```python
from build123d import *

# Parameters (mm, degrees)
EXTRUDE_1_DEPTH     = 6
SKETCH_2_R          = 2
CUT_EXTRUDE_1_DEPTH = 81.380345856


with BuildPart() as part:
    # 草图1 → 凸台-拉伸1 (new body)
    with BuildSketch(Plane(origin=(0, 0, 0), x_dir=(0, 0, -1), z_dir=(1, 0, 0))):
        with BuildLine():
            Line((0, 5), (75, 5))
            ThreePointArc((75, 5), (80, 0), (75, -5))
            Line((75, -5), (0, -5))
            ThreePointArc((0, -5), (-5, 0), (0, 5))
        make_face()
    extrude(amount=EXTRUDE_1_DEPTH)

    # 草图2 → 切除-拉伸1 (cut, through all)
    with BuildSketch(Plane(origin=(6, 0, 0), x_dir=(0, 0, -1), z_dir=(1, 0, 0))):
        with Locations((75, 0)):
            Circle(SKETCH_2_R)
        Circle(SKETCH_2_R)
    extrude(amount=-CUT_EXTRUDE_1_DEPTH, mode=Mode.SUBTRACT)


solid = part.part
```
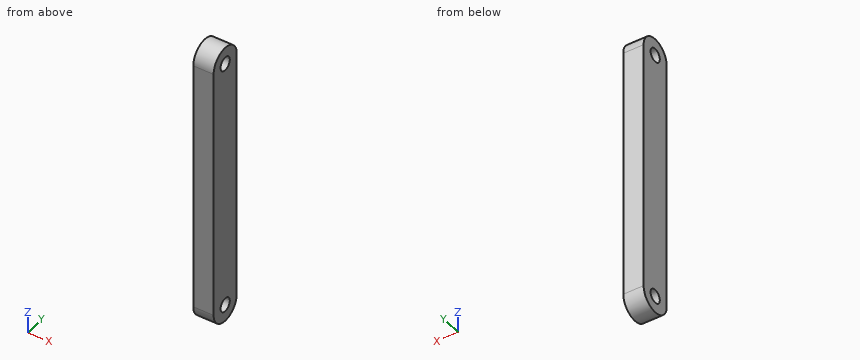
Read the model definition and answer for the solid it produces. Units are mm, in the model's axes. Give positions to 0.01 mm unless a question says otherwise; leave off trailing zeros. Loops run counter-clockwise (first coordinate to the right, second up) from the corner with the lowest first, then second, coordinate; pieces in that order, holes last.
Item 1: Find the intervals of material crossed by line 1 along Y through (x, z) = (2.5, -75); line 2 along Z through (x, y) = (1.4, -1.5); line 3 along Z through (x, y) = (0.3, -0.75), in increasing order.
Item 2: The part is cut by section B-B (x = 3.55). Write down the section's boundary in (y, z).
Item 3: The part is cut by section A-A (y = 0). Write down the section's boundary in (x, z).
Item 4: Each of these flat-tipped pins is pushed along its axis until it touches: pin 1 Ø1.5 at (y, z) = (-0.5, -59.5) entering from -X; pin 2 Ø3 at (y, z) = (0, 0) entering from +X. Where does it stop, or does it pass through?
Taken from the geometry:
1. line 1: y = -5 to -2, 2 to 5
1. line 2: z = -79.77 to -76.32, -73.68 to -1.32, 1.32 to 4.77
1. line 3: z = -79.94 to -76.85, -73.15 to -1.85, 1.85 to 4.94
2. outline: (-5, -75) arc R5 ccw to (5, -75) - (5, 0) arc R5 ccw to (-5, 0) - close; hole circle Ø4 at (0, -75); hole circle Ø4 at (0, 0)
3. outline: (0, -80) - (6, -80) - (6, -77) - (0, -77) - close; (0, -73) - (6, -73) - (6, -2) - (0, -2) - close; (0, 2) - (6, 2) - (6, 5) - (0, 5) - close
4. pin 1: stops at x = 0
4. pin 2: passes through
